Part model, mm, in its own coordinate system. Round coordinates to 2 decimals unless told otherwise and drop trailing zeros. Write each loop counter-clockwise with the first axis right and the second up, starting at its lowest first coordinate (ties: lowest second). Pieces come first, ordered by that corner, then holes.
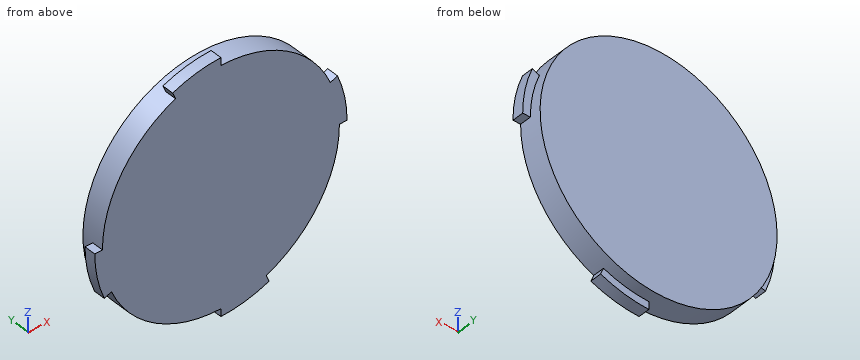
```python
from build123d import *
from build123d.topology import SkipClean

# Parameters (mm, degrees)
SKETCH8_R            = 31
BOSS_EXTRUDE9_DEPTH  = 3
SKETCH11_R           = 31
BOSS_EXTRUDE10_DEPTH = 3


with BuildPart() as part:
    # Sketch8 → Boss-Extrude9 (new body)
    with BuildSketch(Plane(origin=(0, 0, 0), x_dir=(1, 0, 0), z_dir=(0, 1, 0))):
        Circle(SKETCH8_R)
        with BuildLine():
            ThreePointArc((0, -31), (-6.047799982, -30.404343693), (-11.863186403, -28.640265508))
            Line((-11.863186403, -28.640265508), (-12.628553268, -30.488024573))
            ThreePointArc((-12.628553268, -30.488024573), (-6.437980627, -32.365914253), (0, -33))
            Line((0, -33), (0, -31))
        make_face()
        with BuildLine():
            ThreePointArc((-31, 0), (-30.404343693, 6.047799982), (-28.640265508, 11.863186403))
            Line((-28.640265508, 11.863186403), (-30.488024573, 12.628553268))
            ThreePointArc((-30.488024573, 12.628553268), (-32.365914253, 6.437980627), (-33, 0))
            Line((-33, 0), (-31, 0))
        make_face()
        with BuildLine():
            ThreePointArc((12.628553268, 30.488024573), (6.437980627, 32.365914253), (0, 33))
            Line((0, 33), (0, 31))
            ThreePointArc((0, 31), (6.047799982, 30.404343693), (11.863186403, 28.640265508))
            Line((11.863186403, 28.640265508), (12.628553268, 30.488024573))
        make_face()
        with BuildLine():
            Line((33, 0), (31, 0))
            ThreePointArc((31, 0), (30.404343693, -6.047799982), (28.640265508, -11.863186403))
            Line((28.640265508, -11.863186403), (30.488024573, -12.628553268))
            ThreePointArc((30.488024573, -12.628553268), (32.365914253, -6.437980627), (33, 0))
        make_face()
    extrude(amount=BOSS_EXTRUDE9_DEPTH)

    # Sketch11 → Boss-Extrude10 (add)
    with SkipClean():  # the faces are left unmerged after this step: merging them gives an invalid solid
        with BuildSketch(Plane(origin=(0, 3, 0), x_dir=(1, 0, 0), z_dir=(0, 1, 0))):
            with Locations(Location((0, 0, 0), (0, 0, 270))):
                Circle(SKETCH11_R)
        extrude(amount=BOSS_EXTRUDE10_DEPTH)


solid = part.part
```
Q1. Cut at C-C on z = 25. Write the cut outline in (x, y), plus the area to 3 significant figures.
Values follow:
outline: (-18.33, 0) - (18.33, 0) - (18.33, 6) - (-18.33, 6) - close
area: 220 mm2
Q2. Cut at D-D on x = -20. Write the cut outline in (y, z), plus the area to 3 significant figures.
Values follow:
outline: (0, -23.69) - (6, -23.69) - (6, 23.69) - (0, 23.69) - close
area: 284 mm2
Q3. Cut at A-A on y = 1.8. Write the cut outline in (x, z), plus the area to 3 significant figures.
Values follow:
outline: (-33, 0) arc R33 ccw to (-30.49, -12.63) - (-28.64, -11.86) arc R31 ccw to (0, -31) - (0, -33) arc R33 ccw to (12.63, -30.49) - (11.86, -28.64) arc R31 ccw to (31, 0) - (33, 0) arc R33 ccw to (30.49, 12.63) - (28.64, 11.86) arc R31 ccw to (0, 31) - (0, 33) arc R33 ccw to (-12.63, 30.49) - (-11.86, 28.64) arc R31 ccw to (-31, 0) - close
area: 3,120 mm2
Q4. Cut at B-B on x = -4. Write the cut outline in (y, z).
Values follow:
outline: (0, -30.74) - (6, -30.74) - (6, 30.74) - (3, 30.74) - (3, 32.76) - (0, 32.76) - close
Q5. Wall check: L1, parallel to X at y = 1.7, z = 12; L2, parallel to X at y = 4.85, z = 5; L3, parallel to X at y = 5.2, z = -2. Give the ranges that are in metal, low to high.
Values follow:
L1: x = -28.58 to 28.58, 28.97 to 30.74
L2: x = -30.59 to 30.59
L3: x = -30.94 to 30.94
Q6. Drop flat-ended pins along their axis: pin 1 (3 mm diameter, centred on x = -18, y = 5, fed in from +Z); pin 2 (1.3 mm diameter, centred on x = 6, z = -31.5, fed in from +Y); pin 3 (2 mm diameter, centred on y = 2.5, z = 23, fed in from +X). Give the stop position or say it passes through.
Values follow:
pin 1: stops at z = 26.24
pin 2: stops at y = 3
pin 3: stops at x = 21.84
